Can you work these out from the drawing? Everything is in mm from the part's minimum corner. Round coordinates to 2 decimals unless told otherwise and drop trailing zeros. Loops run counter-clockwise (first coordinate to the right, second up) from the corner with the lowest first, then second, coordinate; pieces in that order, holes last. Notation, with made-up numbers: (89, -14.75) - (122, -14.75) arc R17 cw to (122, 11.25) - close; hole circle Ø6 at (62.5, -7). An arc over 180 degrees is marked (long way). Answer as CSV lines item,"result". Start each with the question number.
1) Suppose I cut it at B-B, the plane y = 3.5. Count the separate pieces of the cut face and the enclosed holes in it, then the cut area to 3 significant figures.
2) I'm going to push flat-ended pins straight in: pin 1 Ø1 at (x, y) = (22.5, 3) entering from +Z; pin 2 Ø1.9 at (x, z) = (9.76, 81.51) entering from +Y; pin 3 Ø1.5 at (y, z) = (1.5, 68.5) entering from -X; pin 4 Ø3 at (y, z) = (7, 11.5) entering from -X. Where does each tip first touch, or does it pass through?
3) Please list where these lines run through material, in increasing order: line 1 along Z through (x, y) = (9, 1.5) (1 decimal); line 2 along Z through (x, y) = (58, 1.5); line 3 along Z through (x, y) = (45, 6).
4) Suppose I cut it at C-C, the plane z = 87.5. Write out the boundary of the cut face in (x, y).
5) Suppose I cut it at D-D, the plane x = 25. Write out the boundary of the cut face in (y, z).
6) Suppose I cut it at A-A, the plane x = 55.25. Write out the boundary of the cut face in (y, z) (1 decimal).
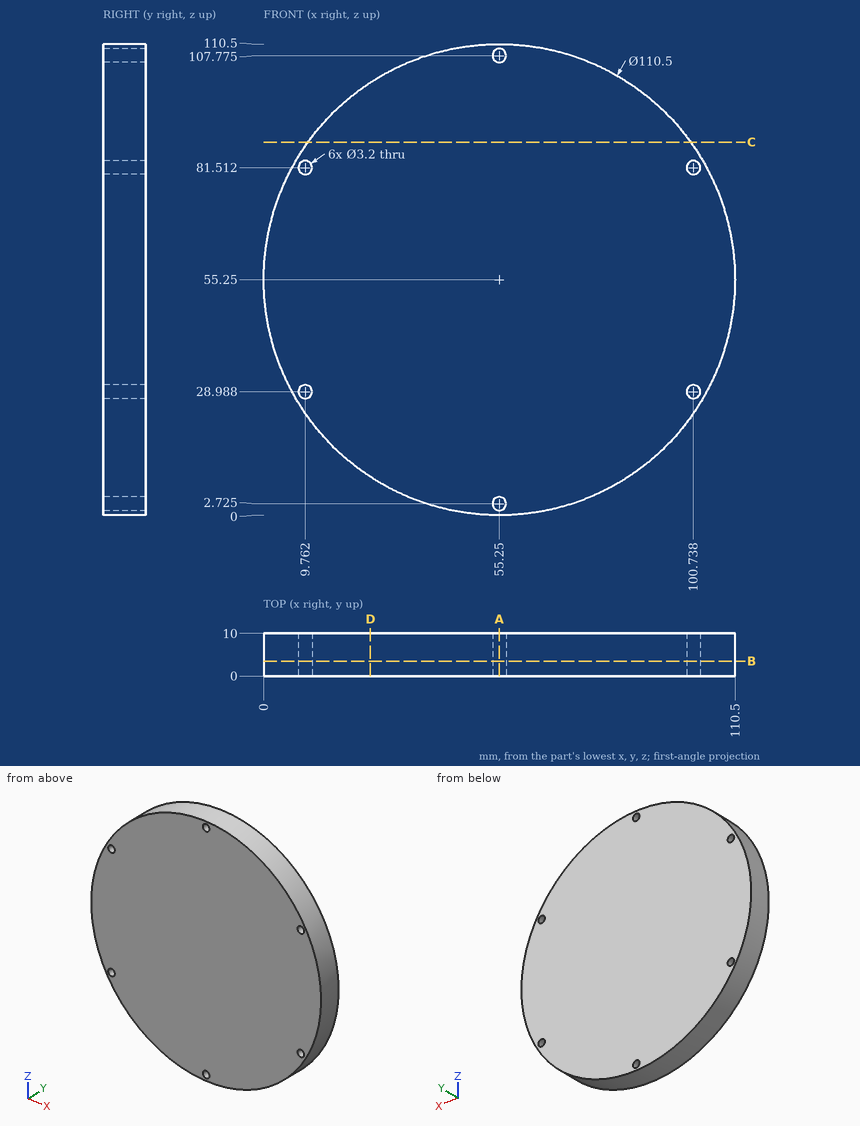
Filled sheet:
1,separate pieces,"1"
1,enclosed holes,"6"
1,area,"9,540 mm²"
2,pin 1,"z = 100.11"
2,pin 2,"through"
2,pin 3,"x = 1.43"
2,pin 4,"x = 19.65"
3,line 1,"25 to 27.6, 30.4 to 80.1, 82.9 to 85.5"
3,line 2,"0.07 to 110.43"
3,line 3,"0.96 to 109.54"
4,outline,"(10.39, 0) - (100.11, 0) - (100.11, 10) - (10.39, 10) - close"
5,outline,"(0, 9.02) - (10, 9.02) - (10, 101.48) - (0, 101.48) - close"
6,outline,"(0, 0) - (10, 0) - (10, 1.1) - (0, 1.1) - close; (0, 4.3) - (10, 4.3) - (10, 106.2) - (0, 106.2) - close; (0, 109.4) - (10, 109.4) - (10, 110.5) - (0, 110.5) - close"
